Build history of the part. All positions in model axes, mm. Face numbers are marked on the shaded views. A direction names the side the tool comes from. Coordinates: 2 decimals unless noted, no trailing zeros. Write each loop counter-clockwise with the first axis right and the second up, starting at its lowest first coordinate (ties: lowest second). Pieces come first, ordered by that corner, then holes. Notation, with made-up numbers: (73, -7) -> (104, -7) arc R19 ccw to (104, 1) -> close; hole circle Ø9 at (-23, 18.25). An arc over 180 degrees is marked (long way). Write each question's results on one line, items separated by ' | '. Start each with the question number.
Q1. Saw through at C-C on y = 6. Give the cut face in (x, z), and give its area (3 significant figures).
Q2. Drill centre lines: line 1 (X direction, y = 15.5, z = -1); line 2 (Z direction, x = -76, y = -62.5); line 3 (Z direction, x = -129, y = 22). Where is each one in solid material? Low to high.
Q3. Saw through at B-B on y = -33. Give the cut face in (x, z).
Q4. Drop flat-ended pins along their axis: pin 1 Ø6 at (x, y) = (-18.5, 7) entering from -Z; pin 2 Ø1.5 at (y, z) = (-29, -4) entering from +X; pin 3 Ø3 at (x, y) = (48, 15) entering from -Z. Give the stop position or say it passes through.
Q5. Tool access for the marked faces 1 and 2: list every direction of +Z, -Z, +X, -X, +Y, -Y with a clear straight run to the whole face (end or side of a thin tool).
from build123d import *

# Parameters (mm, degrees)
BOSS_EXTRUDE1_DEPTH = 168.5
SKETCH2_R           = 3.5
BOSS_EXTRUDE2_DEPTH = 175
FILLET1_R           = 20
SKETCH3_W           = 337
SKETCH3_H           = 35
CUT_EXTRUDE1_DEPTH  = 191.195458673
FILLET2_R           = 10
FILLET3_R           = 5


with BuildPart() as part:
    # Sketch1 → Boss-Extrude1 (new, symmetric)
    with BuildSketch(Plane(origin=(0, 0, 0), x_dir=(0, 0, -1), z_dir=(1, 0, 0))):
        Polygon((-7.5, 73.75), (-7.5, 22.544228634), (3, 4.357695155), (3, -73.75), (7.5, -73.75), (7.5, 5.563466521), (-3, 23.75), (-3, 73.75), align=None)
    extrude(amount=BOSS_EXTRUDE1_DEPTH, both=True)

    # Sketch2 → Boss-Extrude2 (add, symmetric)
    with BuildSketch(Plane(origin=(0, 0, 0), x_dir=(0, 0, -1), z_dir=(1, 0, 0))):
        with Locations((-5.25, 23.147114317)):
            Circle(SKETCH2_R)
    extrude(amount=BOSS_EXTRUDE2_DEPTH, both=True)

    # Fillet1
    fillet1_edges = [part.edges().sort_by_distance(p)[0] for p in [
        (-168.5, 73.75, 5.25),
        (0, 5.563466521, -7.5),
        (0, 4.357695155, -3),
        (168.5, -73.75, -5.25),
        (168.5, 73.75, 5.25),
        (-168.5, -73.75, -5.25),
    ]]
    fillet(fillet1_edges, radius=FILLET1_R)

    # Sketch3 → Cut-Extrude1 (cut, through all)
    with BuildSketch(Plane(origin=(0, 0, 3), x_dir=(-1, 0, 0), z_dir=(0, 0, -1))):
        with Locations((0, 56.25)):
            Rectangle(SKETCH3_W, SKETCH3_H)
    extrude(amount=-CUT_EXTRUDE1_DEPTH, mode=Mode.SUBTRACT)

    # Fillet2
    # the kernel refuses this fillet: 10 mm, written as the material it adds along each edge
    with BuildSketch(Plane(origin=(-168.5, 21.950342364, 1.96096718), x_dir=(0, 0.9916201681580873, -0.12918762364145653), z_dir=(1, 0, 0))) as fillet2_piece_1:
        with BuildLine():
            CenterArc((3.700369944, -9.760226866), FILLET2_R, 102.572148387, 24.85050234)
            Line((-2.376528536, -1.818482419), (0, 0))
            ThreePointArc((0, 0), (0.761840871, -0.083920597), (1.523681742, 0))
        make_face()
    extrude(amount=337)
    with BuildSketch(Plane(origin=(-168.5, 19.700342364, 5.858081497), x_dir=(0, 0.38393032015099443, 0.9233620683506307), z_dir=(1, 0, 0)), Plane(origin=(-168.5, 25.828065641, 3), x_dir=(0, -0.7941744447091721, -0.6076898480070884), z_dir=(1, 0, 0))) as fillet2_piece_2:
        with BuildLine():
            CenterArc((3.700369944, 9.760226866), FILLET2_R, 232.577349272, 24.85050234)
            Line((-2.376528536, 1.818482419), (0, 0))
            ThreePointArc((0, 0), (0.761840871, 0.083920597), (1.523681742, 0))
        make_face()
    extrude(amount=337)
    with BuildSketch(Plane(origin=(-168.5, 25.828065641, 7.5), x_dir=(0, 1, 0), z_dir=(1, 0, 0))) as fillet2_piece_3:
        with BuildLine():
            CenterArc((2.992451535, 10), FILLET2_R, 245.14949766, 24.85050234)
            ThreePointArc((-1.210069101, 0.925925926), (-0.554036856, 0.529610556), (0, 0))
            Line((0, 0), (2.992451535, 0))
        make_face()
    extrude(amount=337)

    # Fillet3
    fillet3_edges = [part.edges().sort_by_distance(p)[0] for p in [
        (-168.5, 38.75, 5.25),
        (168.5, 38.75, 5.25),
    ]]
    fillet(fillet3_edges, radius=FILLET3_R)


solid = part.part
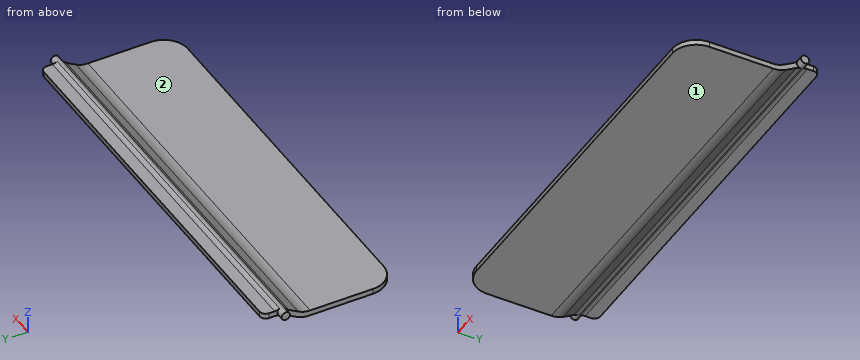
Returned:
1) outline: (-168.5, -6.64) -> (168.5, -6.64) -> (168.5, -1.73) -> (-168.5, -1.73) -> close | area: 1,650 mm2
2) line 1: x = -168.5 to 168.5 | line 2: z = -7.5 to -3 | line 3: z = 1.52 to 8.56
3) outline: (-168.5, -7.5) -> (168.5, -7.5) -> (168.5, -3) -> (-168.5, -3) -> close
4) pin 1: stops at z = -7.14 | pin 2: stops at x = 168.5 | pin 3: stops at z = -2.92
5) face 1: -Z, +X, -X, +Y, -Y | face 2: +Z, +X, -X, -Y
